For this review, take the finished solid that the model builds, in its own axes (mm). Give positions to 0.01 mm unless a question says otherwise; leave off trailing zeros. Order: outer loops, then holes, each group sorted by start corner. A loop starts at its lowest first (then second) coordinate and runs counter-clockwise, first axis right, second up. Notation, with made-up numbers: M 26,15.25 L 63,15.25 A23 cw 63,48.25 Z; hole C 62,82.5 d11. An arc over 180 degrees is marked long. Use CSV: the item, a comma, the result in double quotes. Start each with the question number.
(1) Consider section D-D (y = 2.5). Give the number of separate pieces and of enclosed holes in the cut face, and give its area (3 significant figures).
(2) Wall thickness on L1, parallel to Z at x = -25, y = 0.3; L2, parallel to Z at x = -28.5, y = 1.2; L3, parallel to Z at x = -13.5, y = 0.9: over which ranges is each line inside the solid? List them lowest first. Write a range as from..to.
(3) Clearance check with a flat-ended pin moving along its axis: P1, Ø11, axis at x = 32.5, z = 26.78, coming from the -Y side. State where the tip first meets the part, or that it passes through.
(4) Consider section A-A (z = 0). Write out the cut boundary in (x, y), and give its area (3 significant figures).
(5) Consider section B-B (x = 9). Write out the cut boundary in (y, z).
(6) Consider section C-C (z = 23). Write out the cut boundary in (x, y), and give its area (3 significant figures).
```python
from build123d import *

# Parameters (mm, degrees)
SKETCH1_R           = 32.5
SKETCH1_R_2         = 20
BOSS_EXTRUDE1_DEPTH = 3
SKETCH5_R           = 1.6
CUT_EXTRUDE1_DEPTH  = 10
SKETCH6_R           = 1.65
CUT_EXTRUDE2_DEPTH  = 10
SKETCH8_R           = 6
CUT_EXTRUDE3_DEPTH  = 10


with BuildPart() as part:
    # Sketch1 → Boss-Extrude1 (new body)
    with BuildSketch(Plane(origin=(0, 0, 0), x_dir=(1, 0, 0), z_dir=(0, 1, 0))):
        with BuildLine():
            Line((-42.5, -73.411966665), (-41.810700901, -77.192472856))
            ThreePointArc((-41.810700901, -77.192472856), (0, -112.069134335), (41.810700901, -77.192472856))
            Line((41.810700901, -77.192472856), (42.5, -73.411966665))
            Line((42.5, -73.411966665), (42.5, 36.289181897))
            ThreePointArc((42.5, 36.289181897), (39.241370505, 39.790319974), (35.695303931, 43))
            Line((35.695303931, 43), (-35.695303931, 43))
            ThreePointArc((-35.695303931, 43), (-39.241370505, 39.790319974), (-42.5, 36.289181897))
            Line((-42.5, 36.289181897), (-42.5, -73.411966665))
        make_face()
        with Locations(Location((0, 0, 0), (0, 0, 270))):
            Circle(SKETCH1_R, mode=Mode.SUBTRACT)
        with Locations(Location((0, -69.569134335, 0), (0, 0, 270))):
            Circle(SKETCH1_R_2, mode=Mode.SUBTRACT)
    extrude(amount=BOSS_EXTRUDE1_DEPTH)

    # Sketch5 → Cut-Extrude1 (cut)
    with BuildSketch(Plane(origin=(0, 3, 0), x_dir=(1, 0, 0), z_dir=(0, 1, 0))):
        with Locations(Location((0, -107.069134335, 0), (0, 0, 270))):
            Circle(SKETCH5_R)
    extrude(amount=-CUT_EXTRUDE1_DEPTH, mode=Mode.SUBTRACT)

    # Sketch6 → Cut-Extrude2 (cut)
    with BuildSketch(Plane(origin=(0, 3, 0), x_dir=(1, 0, 0), z_dir=(0, 1, 0))):
        with Locations(Location((-34.5, 35, 0), (0, 0, 270))):
            Circle(SKETCH6_R)
        with Locations(Location((34.5, 35, 0), (0, 0, 270))):
            Circle(SKETCH6_R)
        with Locations(Location((27.5, -34.784567168, 0), (0, 0, 270))):
            Circle(SKETCH6_R)
        with Locations(Location((25.829771931, -81.613754795, 0), (0, 0, 270))):
            Circle(SKETCH6_R)
        with Locations(Location((-25.829771931, -81.613754795, 0), (0, 0, 270))):
            Circle(SKETCH6_R)
        with Locations(Location((-27.5, -34.784567168, 0), (0, 0, 270))):
            Circle(SKETCH6_R)
    extrude(amount=-CUT_EXTRUDE2_DEPTH, mode=Mode.SUBTRACT)

    # Sketch8 → Cut-Extrude3 (cut)
    with BuildSketch(Plane.XZ):
        with Locations(Location((28.5, -29, 0), (0, 0, 270))):
            Circle(SKETCH8_R)
        with Locations(Location((32.5, 26.784567168, 0), (0, 0, 270))):
            Circle(SKETCH8_R)
        with Locations(Location((-32.5, 26.784567168, 0), (0, 0, 90))):
            Circle(SKETCH8_R)
        with Locations(Location((-28.5, -29, 0), (0, 0, 90))):
            Circle(SKETCH8_R)
    extrude(amount=-CUT_EXTRUDE3_DEPTH, mode=Mode.SUBTRACT)


solid = part.part
```
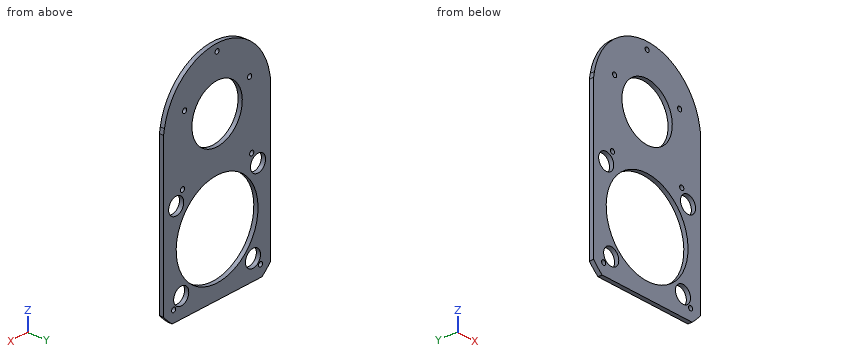
Check result:
1,separate pieces,"1"
1,enclosed holes,"13"
1,area,"7,280 mm^2"
2,L1,"z = -43..-33.87, -24.13..-20.77, 20.77..80.19, 83.04..103.94"
2,L2,"z = -43..-35, -23..-15.62, 15.62..22.31, 31.26..33.47, 36.1..101.1"
2,L3,"z = -43..-29.56, 29.56..54.81, 84.33..109.87"
3,P1,"passes through"
4,outline,"M -42.5,0 L -32.5,0 L -32.5,3 L -42.5,3 Z; M 32.5,0 L 42.5,0 L 42.5,3 L 32.5,3 Z"
4,area,"60.0 mm^2"
5,outline,"M 0,-43 L 3,-43 L 3,-31.23 L 0,-31.23 Z; M 0,31.23 L 3,31.23 L 3,51.71 L 0,51.71 Z; M 0,87.43 L 3,87.43 L 3,111.11 L 0,111.11 Z"
6,outline,"M -42.5,0 L -37.16,0 L -37.16,3 L -42.5,3 Z; M -27.84,0 L -22.96,0 L -22.96,3 L -27.84,3 Z; M 22.96,0 L 27.84,0 L 27.84,3 L 22.96,3 Z; M 37.16,0 L 42.5,0 L 42.5,3 L 37.16,3 Z"
6,area,"61.4 mm^2"
